```python
from build123d import *

# Parameters (mm, degrees)
BOSS_EXTRUDE2_DEPTH = 100
SKETCH2_R           = 5
CUT_EXTRUDE1_DEPTH  = 275.379591078
SKETCH3_R           = 5
CUT_EXTRUDE2_DEPTH  = 10


with BuildPart() as part:
    # Sketch1 → Boss-Extrude2 (new body)
    with BuildSketch(Plane.XY):
        with BuildLine():
            Line((0, 0), (0, 19.6))
            ThreePointArc((0, 19.6), (5.857864376, 33.742135624), (20, 39.6))
            Line((20, 39.6), (204, 39.6))
            Line((204, 39.6), (204, 129.6))
            Line((204, 129.6), (20, 129.6))
            ThreePointArc((20, 129.6), (12.928932188, 126.671067812), (10, 119.6))
            Line((10, 119.6), (10, 100))
            Line((10, 100), (0, 100))
            Line((0, 100), (0, 119.6))
            ThreePointArc((0, 119.6), (5.857864376, 133.742135624), (20, 139.6))
            Line((20, 139.6), (214, 139.6))
            Line((214, 139.6), (214, 29.6))
            Line((214, 29.6), (20, 29.6))
            ThreePointArc((20, 29.6), (12.928932188, 26.671067812), (10, 19.6))
            Line((10, 19.6), (10, 0))
            Line((10, 0), (0, 0))
        make_face()
    extrude(amount=BOSS_EXTRUDE2_DEPTH)

    # Sketch2 → Cut-Extrude1 (cut, through all)
    with BuildSketch(Plane.ZY):
        with Locations((20, 10)):
            Circle(SKETCH2_R)
        with Locations(Location((80, 10, 0), (0, 0, 180))):
            Circle(SKETCH2_R)
    extrude(amount=-CUT_EXTRUDE1_DEPTH, mode=Mode.SUBTRACT)

    # Sketch3 → Cut-Extrude2 (cut)
    with BuildSketch(Plane.ZY):
        with Locations((20, 110)):
            Circle(SKETCH3_R)
        with Locations((80, 110)):
            Circle(SKETCH3_R)
    extrude(amount=-CUT_EXTRUDE2_DEPTH, mode=Mode.SUBTRACT)


solid = part.part
```
The listing builds one solid part. Answer for the finished solid, in the listing's coordinates (mm). A direction names the side the tool comes from. Round coordinates to 2 decimals unless told otherwise and drop trailing zeros. Loops run counter-clockwise (first coordinate to the right, second up) from the corner with the lowest first, then second, coordinate; pieces in that order, holes last. Notation, with made-up numbers: (79, 57.25) - (86, 57.25) arc R23 ccw to (86, 85.25) - close; hole circle Ø3 at (-14, -30.75). An arc over 180 degrees is marked (long way). Return JSON: item names as keys, results as strings. Group by question number.
1. The mould has two halves that part along X. Classify faces 6 (the cylindrical face through (13.01, 126.75, 49.3)), 7 (the flat face through (116, 139.6, 49)), 8 (the flat face through (10, 10, 49)): pulls with the +X half, pulls with the -X half, needs draft (parallel to the pull), parting line crosses it, or undercut.
2. Consider probe 1 along X at (y, z) = (116.5, 17); probe 2 along Y at (x, z) = (42, 85); probe 3 along Y at (x, z) = (4.5, 80). Determine where each line is inside the solid, lowest interval first.
3. The part is cut by section D-D on z = 80. Determine the outline of the cut face in (x, y), then the cut area to 3 significant figures.
4. The part is cut by section B-B on x = 177.5. Determine the outline of the cut face in (y, z), then the cut area to 3 significant figures.
5. Each of these flat-tipped pins is pushed along its axis until it touches: P1, Ø10, axis at y = 5, z = 37, coming from the +X side; P2, Ø6, axis at y = 29.5, z = 33, coming from the -X side; P3, Ø3, axis at x = 4.5, z = 28.5, coming from the -Y side; P4, Ø2, axis at x = 34, z = 40.5, coming from the -Y side. Where does it stop, or does it pass through?
6. Which of the six approach directions +Z, -Z, +X, -X, +Y, -Y give full straight-line access (tool end or side, diameter ignored) to faces 1 (the flat face through (0, 10, 49)), 2 (the flat face through (113, 129.6, 49)), 3 (the cylindrical face through (4.93, 108.085, 84.619)), 4 (the flat face through (118, 29.6, 49)), 5 (the cylindrical face through (5.703, 33.586, 49.3))?
7. The part is cut by section C-C on y = 110. Determine the outline of the cut face in (x, z), then the cut area to 3 significant figures.
8. The part is cut by section A-A on y = 10. Determine the outline of the cut face in (x, z).
Resolved:
{
 "1": {"face 6": "undercut", "face 7": "needs draft", "face 8": "pulls with the +X half"},
 "2": {"probe 1": "x = 0 to 10, 204 to 214", "probe 2": "y = 29.6 to 39.6, 129.6 to 139.6", "probe 3": "y = 0 to 5, 15 to 32.24, 100 to 105, 115 to 132.24"},
 "3": {"outline": "(0, 0) - (10, 0) - (10, 5) - (0, 5) - close; (0, 15) - (10, 15) - (10, 19.6) arc R10 cw to (20, 29.6) - (214, 29.6) - (214, 139.6) - (20, 139.6) arc R20 ccw to (0, 119.6) - (0, 115) - (10, 115) - (10, 119.6) arc R10 cw to (20, 129.6) - (204, 129.6) - (204, 39.6) - (20, 39.6) arc R20 ccw to (0, 19.6) - close; (0, 100) - (10, 100) - (10, 105) - (0, 105) - close", "area": "5,440 mm²"},
 "4": {"outline": "(29.6, 0) - (39.6, 0) - (39.6, 100) - (29.6, 100) - close; (129.6, 0) - (139.6, 0) - (139.6, 100) - (129.6, 100) - close", "area": "2,000 mm²"},
 "5": {"P1": "stops at x = 10", "P2": "stops at x = 1.23", "P3": "stops at y = 0", "P4": "stops at y = 29.6"},
 "6": {"face 1": "+Z, -Z, -X, +Y, -Y", "face 2": "+Z, -Z", "face 3": "-X", "face 4": "+Z, -Z, +X, -Y", "face 5": "+Z, -Z, -X"},
 "7": {"outline": "(0, 0) - (10, 0) - (10, 15) - (0, 15) - close; (0, 25) - (10, 25) - (10, 75) - (0, 75) - close; (0, 85) - (10, 85) - (10, 100) - (0, 100) - close; (204, 0) - (214, 0) - (214, 100) - (204, 100) - close", "area": "1,800 mm²"},
 "8": {"outline": "(0, 0) - (10, 0) - (10, 15) - (0, 15) - close; (0, 25) - (10, 25) - (10, 75) - (0, 75) - close; (0, 85) - (10, 85) - (10, 100) - (0, 100) - close"}
}
